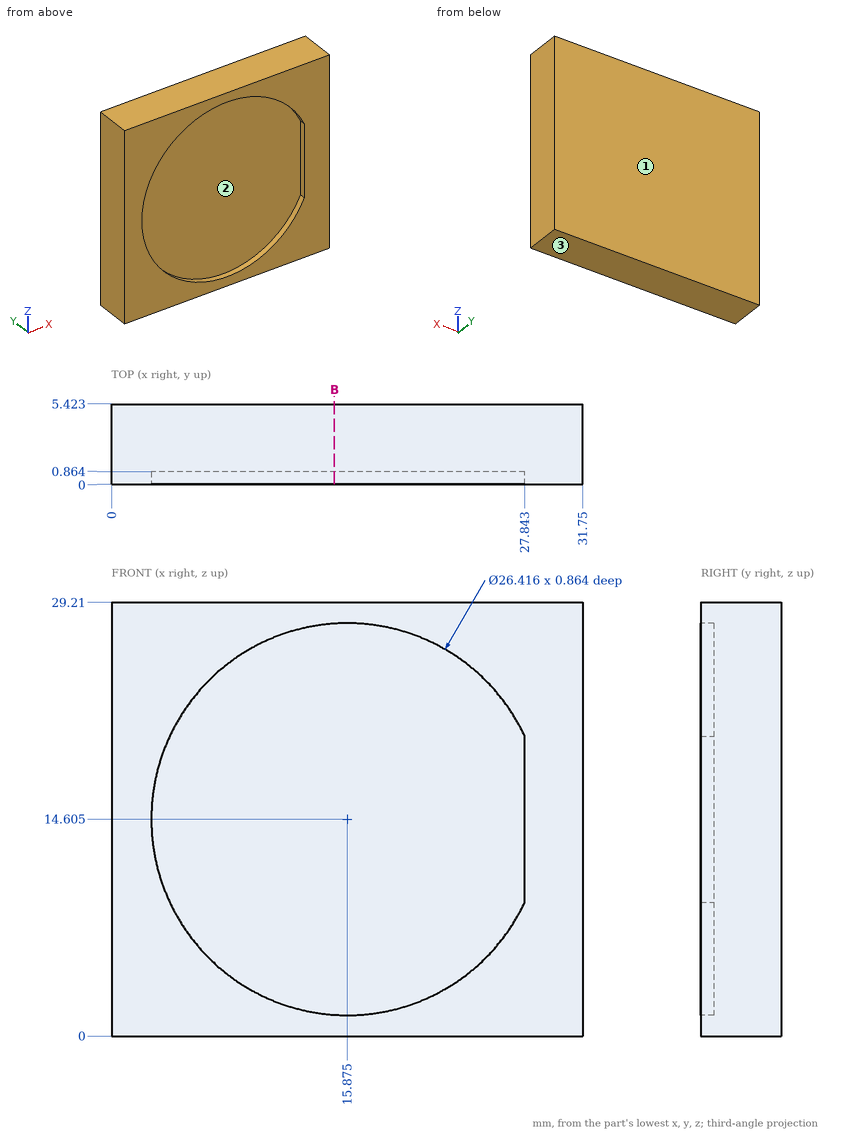
Could you check a few things on this drawing? It's one solid part, dimensions in mm from its lowest x, y, z. Give positions to 0.01 mm unless a question says otherwise; leave off trailing zeros. Order: outer loops, then holes, each group sorted by start corner. A loop starts at its lowest first (then second) coordinate and runs counter-clockwise, first axis right, second up. Notation, with made-up numbers: (-26.75, -31.5) - (-0.75, -31.5) arc R27 ccw to (-0.75, -8.5) - close; hole circle Ø10 at (59, 68). An arc over 180 degrees is marked (long way). Return JSON: item names as keys, results as strings. Group by question number.
Q1. Please list where these lines run through material, in increasing order: line 1 along Y through (x, z) = (7.5, 17); line 2 along Z through (x, y) = (21, 0.55); line 3 along Z through (x, y) = (6.5, 0.65). Write a range as [from, to].
Q2. Thinking about a two-plate mould opening in Z: for the marked faces 1, 2 and 3, which applies, pulls with the +Z half, pulls with the -Z half, needs draft (parallel to the pull), parting line crosses it, or undercut?
Q3. Suppose I cut it at B-B, the plane x = 15. Please give me the cut outline in (y, z), and give its area (3 significant figures).
Q4. Will this pin go through, and if not, where does the flat tip stop? pin 1 Ø7.5 at (x, z) = (14, 12.5) entering from -Y.
Resolved:
{
 "1": {"line 1": "y = [0.86, 5.42]", "line 2": "z = [0, 2.43], [26.78, 29.21]", "line 3": "z = [0, 5.3], [23.91, 29.21]"},
 "2": {"face 1": "needs draft", "face 2": "undercut", "face 3": "pulls with the -Z half"},
 "3": {"outline": "(0, 0) - (5.42, 0) - (5.42, 29.21) - (0, 29.21) - (0, 27.78) - (0.86, 27.78) - (0.86, 1.43) - (0, 1.43) - close", "area": "136 mm2"},
 "4": {"pin 1": "stops at y = 0.86"}
}
